```python
from build123d import *

# Parameters (mm, degrees)
BOSS_EXTRUDE1_DEPTH            = 90
CBORE_FOR_M5_SHCS1_D           = 5.5
CBORE_FOR_M5_SHCS1_CBORE_D     = 10
CBORE_FOR_M5_SHCS1_CBORE_DEPTH = 15


with BuildPart() as part:
    # Sketch2 → Boss-Extrude1 (new, symmetric)
    with BuildSketch(Plane(origin=(0, 0, 0), x_dir=(0, 0, -1), z_dir=(1, 0, 0))):
        Polygon((0, 0), (0, 8), (-65, 14.831775292), (-65, 0), align=None)
    extrude(amount=BOSS_EXTRUDE1_DEPTH, both=True)

    # CBORE for M5 SHCS1 (through all)
    with Locations(Plane(origin=(0, 20, -0.836227706), x_dir=(1, 0, 0), z_dir=(0, 1, 0))):
        with Locations((-50, -45.836227706), (50, -45.836227706)):
            CounterBoreHole(CBORE_FOR_M5_SHCS1_D / 2, CBORE_FOR_M5_SHCS1_CBORE_D / 2, CBORE_FOR_M5_SHCS1_CBORE_DEPTH)


solid = part.part
```
Verification items for the finished model (mm, model axes). A direction names the side the tool comes from. Round coordinates to 2 decimals unless told otherwise and drop trailing zeros. Order: outer loops, then holes, each group sorted by start corner. A loop starts at its lowest first (then second) coordinate and runs counter-clockwise, first axis right, second up. Notation, with made-up numbers: (-28.5, 61) - (-17.5, 61) arc R17 cw to (-17.5, 84) - close; hole circle Ø3 at (24, 63). An arc over 180 degrees is marked (long way). Use CSV: the item, a comma, the result in double quotes. Start each with the question number.
1) Section check D-D, the plane z = 58. Record the cut outline in (x, y).
2) Mould release check, pull along X, two halves, no side actions. Record for faces 3 (the flat face through (-47.8, 5, 47.2)), 4 (the cylindrical face through (-51.08, 9.24, 49.88)), 5 (the flat face through (1, 0, 33)), 6 (the flat face through (90, 6, 33)): +X half, -X half, draft (parallel to the pull), parting line (faces both ways), or undercut.
3) Go/stop test with flat-tipped pins: P1, Ø6, axis at x = -8, z = 29, coming from the +Y side; P2, Ø5, axis at x = -52, z = 47, coming from the +Y side; P3, Ø3, axis at x = 49.5, z = 46, coming from the +Y side; P4, Ø10, axis at x = 45, z = 13, coming from the +Y side. Record where each tip stops, or that it passes through.
4) Section check C-C, the plane x = 13.5. Record the cut outline in (y, z).
5) Access from +Z, -Z, +X, -X, +Y, -Y to the whole of each face (thin tool, end or side, straight path). Record for faces 1 (the cylindrical face through (48.92, 9.24, 49.88)), 2 (the flat face through (1.26, 11.37, 32.05)).
6) Section check B-B, the plane z = 45. Record the cut outline in (x, y).
7) Thickness scan on L1, parallel to X at y = 9.25, z = 45; L2, parallel to X at y = 3.5, z = 45; L3, parallel to Z at x = -50, y = 1.35. Record the ranges inside material, lowest first.
8) Section check A-A, the plane x = -50. Record the cut outline in (y, z).
Answers:
1,outline,"(-90, 0) - (90, 0) - (90, 14.1) - (-90, 14.1) - close"
2,face 3,"undercut"
2,face 4,"undercut"
2,face 5,"draft"
2,face 6,"+X half"
3,P1,"stops at y = 11.36"
3,P2,"stops at y = 13.2"
3,P3,"passes through"
3,P4,"stops at y = 9.89"
4,outline,"(0, 0) - (8, 0) - (14.83, 65) - (0, 65) - close"
5,face 1,"+Y"
5,face 2,"-Z, +X, -X, +Y"
6,outline,"(-90, 0) - (-52.75, 0) - (-52.75, 5) - (-55, 5) - (-55, 12.73) - (-90, 12.73) - close; (-47.25, 0) - (47.25, 0) - (47.25, 5) - (45, 5) - (45, 12.73) - (-45, 12.73) - (-45, 5) - (-47.25, 5) - close; (52.75, 0) - (90, 0) - (90, 12.73) - (55, 12.73) - (55, 5) - (52.75, 5) - close"
7,L1,"x = -90 to -55, -45 to 45, 55 to 90"
7,L2,"x = -90 to -52.75, -47.25 to 47.25, 52.75 to 90"
7,L3,"z = 0 to 42.25, 47.75 to 65"
8,outline,"(0, 0) - (8, 0) - (12.2, 40) - (5, 40) - (5, 42.25) - (0, 42.25) - close; (0, 47.75) - (5, 47.75) - (5, 50) - (13.26, 50) - (14.83, 65) - (0, 65) - close"
